```python
from build123d import *

# Parameters (mm, degrees)
SKETCH1_R                 = 5.5
SKETCH1_R_2               = 2.05
BOSS_EXTRUDE1_DEPTH       = 6
CHAMFER1_SIZE             = 0.5
M4X0_7_TAPPED_HOLE1_D     = 3.3
M4X0_7_TAPPED_HOLE1_DEPTH = 3.5
M4X0_7_TAPPED_HOLE1_TIP   = 0.991420021
CHAMFER2_SIZE             = 0.2


with BuildPart() as part:
    # Sketch1 → Boss-Extrude1 (new body)
    with BuildSketch(Plane.XY):
        Circle(SKETCH1_R)
        Circle(SKETCH1_R_2, mode=Mode.SUBTRACT)
    extrude(amount=BOSS_EXTRUDE1_DEPTH)

    # Chamfer1
    chamfer1_edges = [part.edges().sort_by_distance(p)[0] for p in [
        (-2.05, 0, 0),
        (-2.05, 0, 6),
    ]]
    chamfer(chamfer1_edges, length=CHAMFER1_SIZE)

    # M4x0.7 Tapped Hole1
    with Locations(Plane(origin=(0.156712009, -5.497766942, 2.924685325), x_dir=(-0.999593989, -0.028493093, 0), z_dir=(0.028493093, -0.999593989, 0))):
        with Locations((0, 0)):
            Hole(M4X0_7_TAPPED_HOLE1_D / 2, depth=M4X0_7_TAPPED_HOLE1_DEPTH)
            with Locations((0, 0, -(M4X0_7_TAPPED_HOLE1_DEPTH + M4X0_7_TAPPED_HOLE1_TIP / 2))):  # 118° drill point
                Cone(0, M4X0_7_TAPPED_HOLE1_D / 2, M4X0_7_TAPPED_HOLE1_TIP, mode=Mode.SUBTRACT)

    # Chamfer2
    chamfer2_edges = [part.edges().sort_by_distance(p)[0] for p in [
        (-5.5, 0, 0),
        (-5.5, 0, 6),
    ]]
    chamfer(chamfer2_edges, length=CHAMFER2_SIZE)


solid = part.part
```
Model file for the job. Use its own axes, mm. A direction names the side the tool comes from. Coordinates: 2 decimals unless noted, no trailing zeros. Write each loop counter-clockwise with the first axis right and the second up, starting at its lowest first coordinate (ties: lowest second). Pieces come first, ordered by that corner, then holes. Notation, with made-up numbers: (23, 17) - (44, 17) arc R20 cw to (44, 53) - close; hole circle Ø1 at (85.5, -17.5). An arc over 180 degrees is marked (long way). One line per item, written item: value. Start each with the question number.
1. Slice it at C-C (x = 0). Count the separate pieces of the cut face and the enclosed holes in it, plus the area to 3 significant figures.
2. Mould opens along Y. For faces 3 (the cylindrical face through (-0.267, 2.033, 2.965)), 4 (the conical face through (1.34, -1.746, 2.901)), 5 (the cylindrical face through (-0.716, 5.453, 2.961)) say: released by +Y, released by -Y, zero draft, split by the parting line, or undercut.
3. Tool access for faces 1 (the flat face through (-1.3, 2.4, 0)), 2 (the conical face through (-1.24, -1.82, 2.95)): list every direction of +Z, -Z, +X, -X, +Y, -Y with a clear straight run to the whole face (end or side of a thin tool).
4. Flat gauge pins, fed straight in: pin 1 (1.5 mm diameter, centred on x = 3, z = 2, fed in from -Y); pin 2 (2 mm diameter, centred on x = 0, y = 2, fed in from -Z); pin 3 (1.5 mm diameter, centred on y = -1, z = 3.5, fed in from +X); pin 4 (1 mm diameter, centred on x = -2.5, z = 3.5, fed in from +Y). Where does each tip first touch, or does it go through?
5. Probe line 1 (Y direction, x = 0, z = 2.95); line 2 (Z direction, x = 1.5, y = -3); line 3 (X direction, y = -4.5, z = 2.3). List the from-to ranges inside material, lowest first. Write a range as from..to.
6. Slice it at A-A (y = 0). Write the cut outline in (x, z), plus the area to 3 significant figures.
7. Slice it at B-B (z = 1). Write the cut outline in (x, y), plus the area to 3 significant figures.
Answers below:
1. separate pieces: 3
1. enclosed holes: 0
1. area: 29.5 mm^2
2. face 3: undercut
2. face 4: released by -Y
2. face 5: split by the parting line
3. face 1: -Z, +X, -X, +Y, -Y
3. face 2: none
4. pin 1: stops at y = -5.02
4. pin 2: stops at z = 0
4. pin 3: stops at x = 5.49
4. pin 4: stops at y = 5.12
5. line 1: y = 2.05..5.5
5. line 2: z = 0..2.07, 3.78..6
5. line 3: x = -3.16..-1.4, 1.66..3.16
6. outline: (-5.5, 0.2) - (-5.3, 0) - (-2.55, 0) - (-2.05, 0.5) - (-2.05, 5.5) - (-2.55, 6) - (-5.3, 6) - (-5.5, 5.8) - close; (2.05, 0.5) - (2.55, 0) - (5.3, 0) - (5.5, 0.2) - (5.5, 5.8) - (5.3, 6) - (2.55, 6) - (2.05, 5.5) - close
6. area: 40.8 mm^2
7. outline: circle Ø11 at (0, 0); hole circle Ø4.1 at (0, 0)
7. area: 81.8 mm^2
